The listing builds one solid part. Answer for the finished solid, in the listing's coordinates (mm). Face numbers are marked on the shaded views. Give positions to 0.01 mm unless a question says otherwise; leave off trailing zeros. Write each loop counter-clockwise with the first axis right and the second up, starting at its lowest first coordinate (ties: lowest second). Pieces come first, ordered by that corner, then holes.
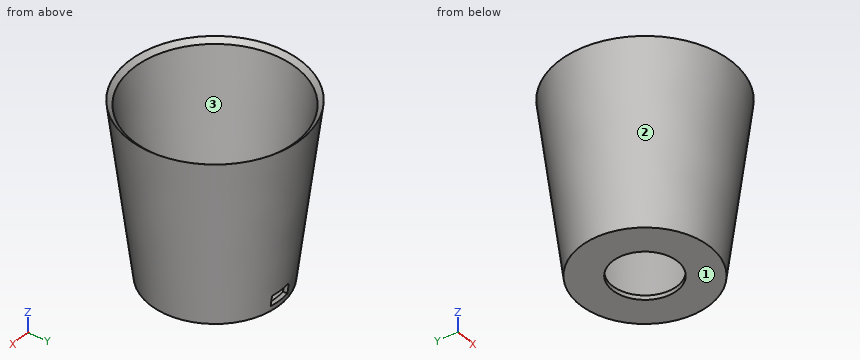
```python
from build123d import *

# Parameters (mm, degrees)
F2_R     = 50.8
F0_R     = 38.1
F4_T     = -2.54
F5_W     = 12.7
F5_H     = 6.35
F6_DEPTH = 40.132
F8_R     = 19.05
F9_DEPTH = 25.4


# Not quite as in the source:
# - a fillet or chamfer that OpenCascade refuses, or shapes differently, is made with other operations: its cross-section is extruded or revolved along the edge and cut away or added


with BuildPart() as f3:
    # F2 (on offset) → F3 section 0
    with BuildSketch(Plane.XY.offset(101.6)):
        Circle(F2_R)
    # F0 (on Top) → F3 section 1
    with BuildSketch(Plane.XY):
        Circle(F0_R)
    loft()

    # F4
    f4_openings = [f3.faces().sort_by_distance(p)[0] for p in [
        (0, 0, 101.6),
    ]]
    offset(amount=F4_T, openings=f4_openings, kind=Kind.INTERSECTION)

    # F5 (on Front) → F6 (cut)
    with BuildSketch(Plane.XZ):
        with Locations((0, 6.35)):
            Rectangle(F5_W, F5_H)
    extrude(amount=-F6_DEPTH, mode=Mode.SUBTRACT)

    # F7: chamfer of 2.54 on 1 edges, made by hand

    # F7_s1 → F7_t2 (revolve, cut)
    with BuildSketch(Plane.XZ):
        Polygon((50.7802331649, 101.6), (47.9251849391, 99.0796141931), (48.2402331649, 101.6), align=None)
    revolve(axis=Axis((0, 0, 101.6), (0, 0, -1)), mode=Mode.SUBTRACT)

    # F8 (on face) → F9 (cut)
    with BuildSketch(Plane.XY.offset(2.54)):
        Circle(F8_R)
    extrude(amount=-F9_DEPTH, mode=Mode.SUBTRACT)


solid = f3.part
```
Item 1: A cutting plane is placed at A-A, the plane x = 0. Give the vertices of the cut face in (y, z) (3 decimals), plus the area to 3 significant figures.
Conclusion:
outline: (-50.8, 101.6) - (-38.1, 0) - (-19.05, 0) - (-19.05, 2.54) - (-35.858, 2.54) - (-47.925, 99.08) - (-50.78, 101.6) - close; (19.05, 0) - (38.1, 0) - (38.497, 3.175) - (35.937, 3.175) - (35.858, 2.54) - (19.05, 2.54) - close; (36.731, 9.525) - (39.291, 9.525) - (50.8, 101.6) - (50.78, 101.6) - (47.925, 99.08) - close
area: 582 mm2
Item 2: Consider probe 1 along Z at (x, y) = (-25.5, -12); probe 2 along Y at (x, z) = (6, 14); probe 3 along Y at (x, z) = (0, 1) (3 decimals). Determine where each line is inside the solid, lowest interval first.
Conclusion:
probe 1: z = 0 to 2.54
probe 2: y = -39.4 to -36.8, 36.8 to 39.4
probe 3: y = -38.225 to -19.05, 19.05 to 38.225
Item 3: Each of these flat-tipped pins is pushed along its axis until it touches: P1, Ø0.9, axis at x = 2.5, y = 38, coming from the -Z side; P2, Ø8, axis at x = 24, z = 38, coming from the -Y side; P3, Ø3, axis at x = -14, z = 37.5, coming from the -Y side; P4, Ø1, axis at x = 27.5, z = 59, coming from the +Y side. Where does it stop, or does it pass through?
Conclusion:
P1: stops at z = 0
P2: stops at y = -37.97
P3: stops at y = -40.96
P4: stops at y = 36.6
Item 4: A cutting plane is placed at C-C, the plane z = 49.5. Give the vertices of the cut face in (x, y) (1 decimal), plus the area to 3 significant figures.
Conclusion:
outline: circle Ø88.6 at (0, 0); hole circle Ø83.5 at (0, 0)
area: 692 mm2
Item 5: A cutting plane is placed at B-B, the plane z = 84. Give the vertices of the cut face in (x, y), plus the area to 3 significant figures.
Conclusion:
outline: circle Ø97.2 at (0, 0); hole circle Ø92.08 at (0, 0)
area: 761 mm2
Item 6: Determine the mould class of the marked faces 1, 2 and 3 for opening direction X: pulls with the +X half, pulls with the -X half, needs draft (parallel to the pull), parting line crosses it, or undercut.
Conclusion:
face 1: needs draft
face 2: parting line crosses it
face 3: undercut
